The drawing under review shows one solid part. Ordinate dimensions are in mm from its lowest x, y, z. A direction names the side the tool comes from. Coordinates: 2 decimals unless noted, no trailing zeros. Write each loop counter-clockwise with the first axis right and the second up, starting at its lowest first coordinate (ties: lowest second). Pieces come first, ordered by that corner, then holes. Notation, with made-up numbers: (-6.75, 28) -> (8.25, 28) arc R13 ccw to (8.25, 39) -> close; hole circle Ø6 at (-11.75, 73.25). An arc over 180 degrees is marked (long way). Put each result on its own line as item: value. Start each with the question number.
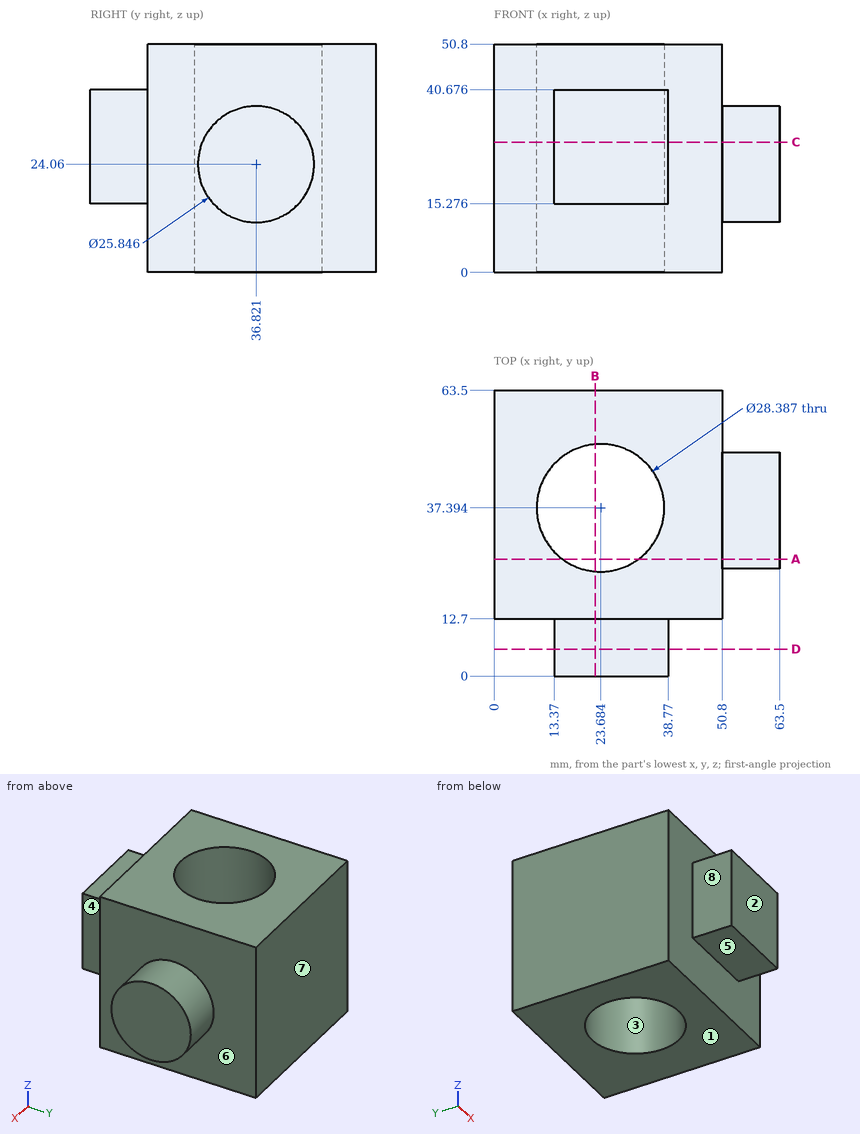
1. Consider section D-D on y = 6. State the section outline as (x, z) points, then the cut area to 3 significant figures.
2. Consider section A-A on y = 26. State the section outline as (x, z) points (1 decimal), then the cut area to 3 significant figures.
3. Consider section B-B on x = 22.5. State the section outline as (y, z) points.
4. Consider section C-C on z = 29. State the section outline as (x, y) points (1 decimal), then the cut area to 3 significant figures.
5. Tool access review of the marked faces 4, 5, 6, 7 and 8: name each direction out of +Z, -Z, +X, -X, +Y, -Y from which nothing blocks a thin tool from reaching the whole face with its end or side.
6. The part is to be moulded in two halves that separate along Y. For the marked faces 1, 2 and 3, say which applies: released by +Y, released by -Y, zero draft, split by the parting line, or undercut.
7. Wall thickness on line 1 (X direction, y = 37, z = 29); line 2 (Y direction, x = 5, z = 37); line 3 (X direction, y = 54, z = 30.5): over which ranges is each line inside the solid? List them lowest first. Write a range as from..to.
8. Insertion check: P1, Ø6.5, axis at y = 6, z = 34, coming from the +X side; P2, Ø10, axis at x = 24.5, y = 7.5, coming from the -Z side; P3, Ø5, axis at y = 38.5, z = 39.5, coming from the +X side. Each pin has a flat end and moves straight along its axis. Give the tip position at first contact, or say it passes through.
Output values:
1. outline: (13.37, 15.28) -> (38.77, 15.28) -> (38.77, 40.68) -> (13.37, 40.68) -> close
1. area: 645 mm^2
2. outline: (0, 0) -> (15.2, 0) -> (15.2, 50.8) -> (0, 50.8) -> close; (32.1, 0) -> (50.8, 0) -> (50.8, 17) -> (63.5, 17) -> (63.5, 31.1) -> (50.8, 31.1) -> (50.8, 50.8) -> (32.1, 50.8) -> close
2. area: 1,900 mm^2
3. outline: (0, 15.28) -> (12.7, 15.28) -> (12.7, 0) -> (23.25, 0) -> (23.25, 50.8) -> (12.7, 50.8) -> (12.7, 40.68) -> (0, 40.68) -> close; (51.54, 0) -> (63.5, 0) -> (63.5, 50.8) -> (51.54, 50.8) -> close
4. outline: (0, 12.7) -> (13.4, 12.7) -> (13.4, 0) -> (38.8, 0) -> (38.8, 12.7) -> (50.8, 12.7) -> (50.8, 24.9) -> (63.5, 24.9) -> (63.5, 48.8) -> (50.8, 48.8) -> (50.8, 63.5) -> (0, 63.5) -> close; hole circle Ø28.4 at (23.7, 37.4)
4. area: 2,570 mm^2
5. face 4: +Z, -Z, +X, -Y
5. face 5: -Z, +X, -X, -Y
5. face 6: +X
5. face 7: +Z, -Z, +X, -X, +Y
5. face 8: +Z, -Z, -X, -Y
6. face 1: zero draft
6. face 2: released by -Y
6. face 3: undercut
7. line 1: x = 0..9.5, 37.87..63.5
7. line 2: y = 12.7..63.5
7. line 3: x = 0..50.8
8. P1: stops at x = 38.77
8. P2: stops at z = 15.28
8. P3: stops at x = 50.8
